```python
from build123d import *

# Parameters (mm, degrees)
SKETCH1_R                    = 7
SKETCH1_R_2                  = 0.975
BOSS_EXTRUDE1_DEPTH          = 5
SKETCH3_R                    = 3.075
CUT_EXTRUDE1_DEPTH           = 5
SKETCH4_R                    = 0.775
BOSS_EXTRUDE3_DEPTH          = 1.5
CHAMFER1_SIZE                = 0.3
CIRPATTERN1_COUNT            = 4
CHAMFER1_OF_CIRPATTERN1_SIZE = 0.3
SKETCH8_R                    = 0.4
CHAMFER2_SIZE                = 0.4


with BuildPart() as part:
    # Sketch1 → Boss-Extrude1 (new, symmetric)
    with BuildSketch(Plane(origin=(0, 0, 0), x_dir=(1, 0, 0), z_dir=(0, 1, 0))):
        with Locations(Location((0, 0, 0), (0, 0, 270))):
            Circle(SKETCH1_R)
        with Locations(Location((0, 0, 0), (0, 0, 270))):
            Circle(SKETCH1_R_2, mode=Mode.SUBTRACT)
    extrude(amount=BOSS_EXTRUDE1_DEPTH, both=True)

    # Sketch3 → Cut-Extrude1 (cut)
    with BuildSketch(Plane(origin=(0, 5, 0), x_dir=(1, 0, 0), z_dir=(0, 1, 0))):
        with Locations(Location((0, 0, 0), (0, 0, 270))):
            Circle(SKETCH3_R)
    extrude(amount=-CUT_EXTRUDE1_DEPTH, mode=Mode.SUBTRACT)

    # Sketch4 → Boss-Extrude3 (add)
    with BuildSketch(Plane.XZ.offset(-5)):
        with Locations(Location((4.5, 0, 0), (0, 0, 270))):
            Circle(SKETCH4_R)
    boss_extrude3 = extrude(amount=-BOSS_EXTRUDE3_DEPTH)

    # Chamfer1
    chamfer1_edges = [part.edges().sort_by_distance(p)[0] for p in [
        (4.5, 6.5, 0.775),
    ]]
    chamfer(chamfer1_edges, length=CHAMFER1_SIZE)

    # CirPattern1: Boss-Extrude3 ×4 about axis
    cirpattern1_axis = Axis((0, 0, 0), (0, 1, 0))
    for i in range(1, CIRPATTERN1_COUNT):
        add(boss_extrude3.rotate(cirpattern1_axis, i * 360 / CIRPATTERN1_COUNT))

    # Chamfer1 of CirPattern1
    chamfer1_of_cirpattern1_edges = [part.edges().sort_by_distance(p)[0] for p in [
        (0.775, 6.5, -4.5),
        (-4.5, 6.5, -0.775),
        (-0.775, 6.5, 4.5),
    ]]
    chamfer(chamfer1_of_cirpattern1_edges, length=CHAMFER1_OF_CIRPATTERN1_SIZE)

    # Sketch8 → Cut-Revolve1 (revolve, cut)
    with BuildSketch(Plane.XY, mode=Mode.PRIVATE) as cut_revolve1_sk:
        with Locations((7, 1)):
            Circle(SKETCH8_R)
    revolve(cut_revolve1_sk.sketch.rotate(Axis((0, 0, 0), (0, 1, 0)), 90), axis=Axis((0, 0, 0), (0, 1, 0)), mode=Mode.SUBTRACT)

    # Chamfer2
    chamfer2_edges = [part.edges().sort_by_distance(p)[0] for p in [
        (0, -5, -7),
        (0, 5, -7),
    ]]
    chamfer(chamfer2_edges, length=CHAMFER2_SIZE)


solid = part.part
```
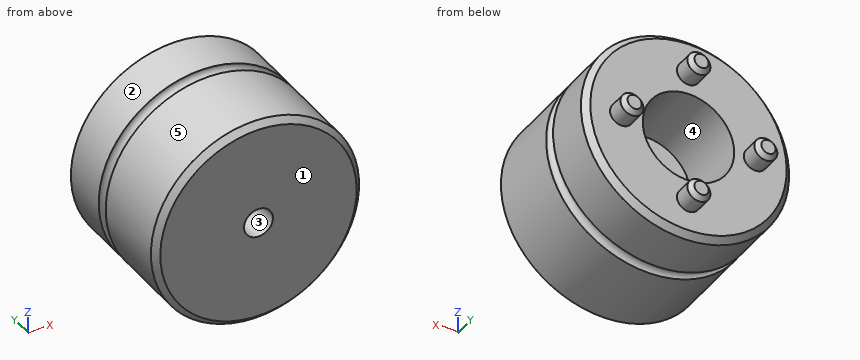
Can you work these out from the model? Positions are in its coordinate system, mm. Face numbers are marked on the shaded views. A direction names the side the tool comes from. Give positions to 0.01 mm unless a question says otherwise; leave off trailing zeros. Loops run counter-clockwise (first coordinate to the right, second up) from the corner with the lowest first, then second, coordinate; pieces in that order, holes last. Notation, with made-up numbers: M 89,85.25 L 106,85.25 A16 ccw 106,116.25 Z; hole C 63,87 d6. An arc over 180 degrees is marked long. Use one line per item in the form item = value. Start each with the question number.
(1) Please list where these lines run through material, in increasing order: line 1 (X direction, y = 1.55, z = 0) (3 decimals); line 2 (X direction, y = -1.5, z = 0) (3 decimals); line 3 (Y direction, x = -4.75, z = 1.5).
(2) I want a section at C-C, the plane y = 5.25. Write out the boundary of the cut face in (x, z) (3 decimals).
(3) On a 3-axis mill with a long thin cutter (end or side, diameter ignored), from which of +Z, -Z, +X, -X, +Y, -Y can I reach the whole of each face in a straight line? I mean the marked faces 4 and 5. Say none if no direction works.
(4) Thinking about a two-plate mould opening in Z: for the marked faces 1, 2 and 3, which applies, released by +Z, released by -Z, zero draft, split by the parting line, or undercut?
(5) I'm going to push flat-ended pins straight in: P1, Ø3, axis at x = 0, z = 0, coming from the +Y side; P2, Ø5, axis at y = 1.5, z = -4, coming from the -X side; P3, Ø3, axis at x = 5, y = -1.5, coming from the -Z side. Where does each tip first touch, or does it pass through?
(6) I want a section at D-D, the plane y = -1.5. Write out the boundary of the cut face in (x, z) (3 decimals).
Worked out:
q1.line_1 = -7 to -3.075, 3.075 to 7
q1.line_2 = -7 to -0.975, 0.975 to 7
q1.line_3 = -5 to 5
q2.outline = C -4.5,0 d1.55; C 0,-4.5 d1.55; C 0,4.5 d1.55; C 4.5,0 d1.55
q3.face_4 = +Y
q3.face_5 = +Y, -Y
q4.face_1 = zero draft
q4.face_2 = split by the parting line
q4.face_3 = undercut
q5.P1 = 0
q5.P2 = -6.84
q5.P3 = -6.06
q6.outline = C 0,0 d14; hole C 0,0 d1.95
